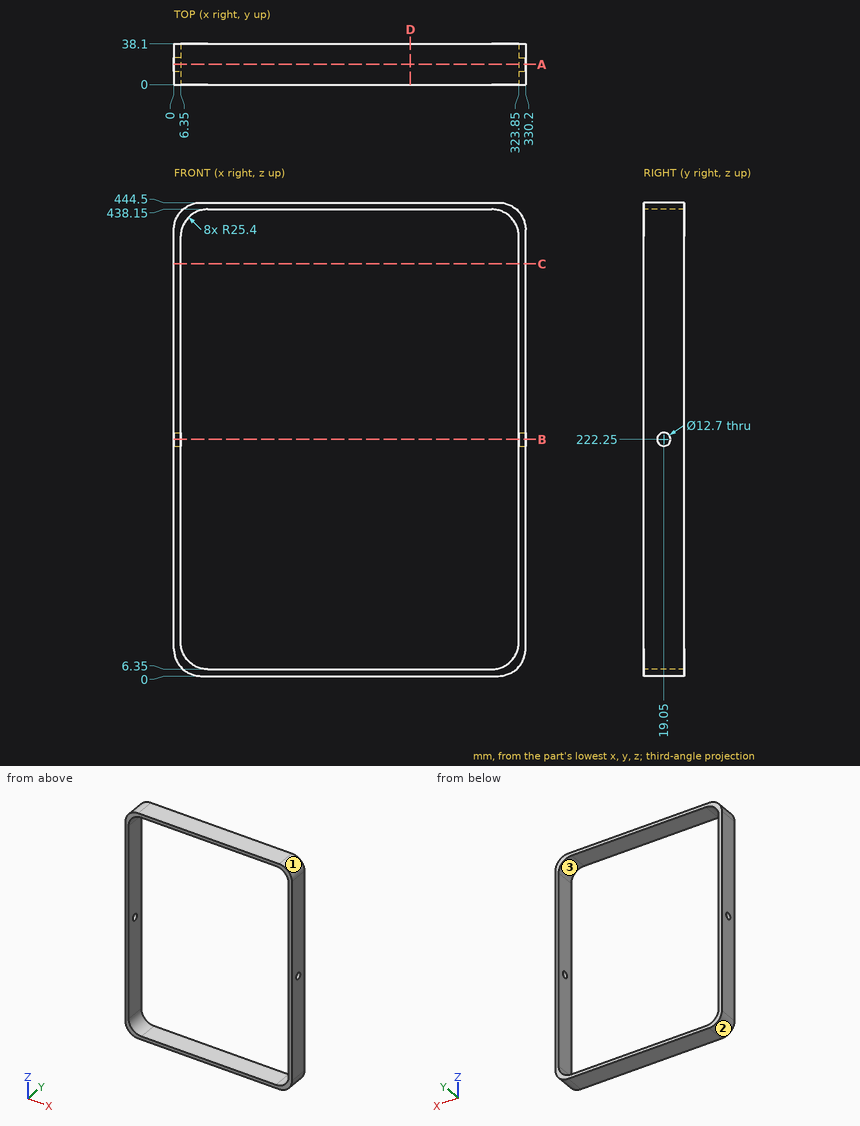
Print and shaded views of the part. All mm, measured from the part's lowest x, y and z. Coordinates: 2 decimals unless noted, no trailing zeros. Loops run counter-clockwise (first coordinate to the right, second up) from the corner with the lowest first, then second, coordinate; pieces in that order, holes last. Notation, with made-up numbers: (15.25, -18.75) -> (19.25, -18.75) arc R23 cw to (19.25, 20.25) -> close; hole circle Ø1 at (13, 14.25). An arc over 180 degrees is marked (long way). Use a Markdown table: item, result. Add a question column.
Item 1: Band-saw the part on A-A on y = 19.05. Write the cut outline in (x, z).
Item 2: Band-saw the part on D-D on x = 222. Write the cut outline in (y, z).
Item 3: Pull direction Z, two halves, no side cores. Call the marked faces 1, 2 and 3: +Z half, -Z half, draft (parallel to the pull), parting line (faces both ways), or undercut.
Item 4: Band-saw the part on C-C on z = 387. Write the cut outline in (x, y).
Item 5: Probe probe 1 along Z at (x, y) = (199, 8.5); probe 2 along X at (y, z) = (5, 135); probe 3 along Y at (x, z) = (3, 222). List the from-to ranges inside material, lowest first.
Item 6: Band-saw the part on B-B on z = 222.25. Write the cut outline in (x, y).
Geometry says:
| question | item | result |
|---|---|---|
| 1 | outline | (0, 25.4) arc R25.4 ccw to (25.4, 0) -> (304.8, 0) arc R25.4 ccw to (330.2, 25.4) -> (330.2, 215.9) -> (323.85, 215.9) -> (323.85, 31.75) arc R25.4 cw to (298.45, 6.35) -> (31.75, 6.35) arc R25.4 cw to (6.35, 31.75) -> (6.35, 215.9) -> (0, 215.9) -> close; (0, 228.6) -> (6.35, 228.6) -> (6.35, 412.75) arc R25.4 cw to (31.75, 438.15) -> (298.45, 438.15) arc R25.4 cw to (323.85, 412.75) -> (323.85, 228.6) -> (330.2, 228.6) -> (330.2, 419.1) arc R25.4 ccw to (304.8, 444.5) -> (25.4, 444.5) arc R25.4 ccw to (0, 419.1) -> close |
| 2 | outline | (0, 0) -> (38.1, 0) -> (38.1, 6.35) -> (0, 6.35) -> close; (0, 438.15) -> (38.1, 438.15) -> (38.1, 444.5) -> (0, 444.5) -> close |
| 3 | face 1 | +Z half |
| 3 | face 2 | -Z half |
| 3 | face 3 | undercut |
| 4 | outline | (0, 0) -> (6.35, 0) -> (6.35, 38.1) -> (0, 38.1) -> close; (323.85, 0) -> (330.2, 0) -> (330.2, 38.1) -> (323.85, 38.1) -> close |
| 5 | probe 1 | 0 to 6.35, 438.15 to 444.5 |
| 5 | probe 2 | 0 to 6.35, 323.85 to 330.2 |
| 5 | probe 3 | 0 to 12.7, 25.4 to 38.1 |
| 6 | outline | (0, 0) -> (6.35, 0) -> (6.35, 12.7) -> (0, 12.7) -> close; (0, 25.4) -> (6.35, 25.4) -> (6.35, 38.1) -> (0, 38.1) -> close; (323.85, 0) -> (330.2, 0) -> (330.2, 12.7) -> (323.85, 12.7) -> close; (323.85, 25.4) -> (330.2, 25.4) -> (330.2, 38.1) -> (323.85, 38.1) -> close |
